Part model, mm, in its own coordinate system. Face numbers are marked on the shaded views. A direction names the side the tool comes from. Round coordinates to 2 decimals unless told otherwise and drop trailing zeros. Write each loop counter-clockwise with the first axis right and the second up, starting at its lowest first coordinate (ties: lowest second). Pieces come first, ordered by that corner, then holes. Notation, with made-up numbers: M 23.5,-11 L 52.5,-11 A27 ccw 52.5,16 Z; hole C 59,80.5 d2. An arc over 180 degrees is marked long. One line per question, with ' | ' between items. Start each with the question number.
1) Drop flat-ended pins along their axis: pin 1 Ø1.5 at (y, z) = (4.5, 2.5) entering from +X; pin 2 Ø0.7 at (y, z) = (-5, 1.5) entering from +X; pin 3 Ø1 at (x, y) = (2.5, -0.5) entering from -Z. Give the stop position or say it passes through.
2) Mould opens along Y. For the marked faces 1, 2, 3 and 4 say: pulls with the +Y half, pulls with the -Y half, needs draft (parallel to the pull), parting line crosses it, or undercut.
3) Saw through at A-A (z = 1.3). List the corners of the cut face in (x, y) (3 decimals), plus the area to 3 significant figures.
4) Saw through at B-B (z = 2.4). List the corners of the cut face in (x, y) (3 decimals), plus the area to 3 significant figures.
5) Wall check: probe 1 along Y at (x, z) = (4.5, 2.75); probe 2 along X at (y, z) = (-0.5, 3.05); probe 3 along Y at (x, z) = (-0.75, 3.2). Give the ranges that are in metal, low to high. Write a range as [from, to].
6) Saw through at D-D (z = 0.25). List the corners of the cut face in (x, y) (3 decimals), plus the area to 3 significant figures.
7) Tool access for the marked faces 5, 6, 7 and 8: list every direction of +Z, -Z, +X, -X, +Y, -Y with a clear straight run to the whole face (end or side of a thin tool).
8) Saw through at C-C (x = 5). List the corners of the cut face in (y, z), plus the area to 3 significant figures.
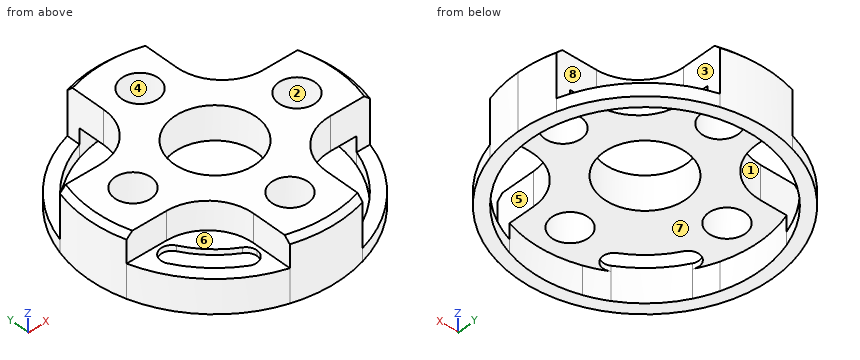
```python
from build123d import *
from build123d import SkipClean  # not in build123d's __all__

# Parameters (mm, degrees)
F0_R     = 1
F0_R_2   = 2.25
F1_DEPTH = 3.4
F2_DEPTH = 0.7
F3_DEPTH = 1.85
F4_DEPTH = 1.55
F5_R     = 2.5
F6_SIZE  = 0.3
F8_DEPTH = 1.851


# Not quite as in the source:
# - after a boolean that leaves OpenCascade's solid faulty, fix() repairs it


with BuildPart() as f1:
    # F0 (on Top) → F1 (new body)
    with BuildSketch(Plane.XY):
        with BuildLine():
            Line((2, 5.9477411679), (2, 6.6821123157))
            ThreePointArc((2, 6.6821123157), (0, 6.975), (-2, 6.6821123157))
            Line((-2, 6.6821123157), (-2, 5.9477411679))
            ThreePointArc((-2, 5.9477411679), (0, 6.275), (2, 5.9477411679))
        make_face()
        with BuildLine():
            ThreePointArc((6.275, 0), (6.1926448642, 1.013298863), (5.9477411679, 2))
            Line((5.9477411679, 2), (2, 2))
            Line((2, 2), (2, 5.9477411679))
            ThreePointArc((2, 5.9477411679), (0, 6.275), (-2, 5.9477411679))
            Line((-2, 5.9477411679), (-2, 2))
            Line((-2, 2), (-5.9477411679, 2))
            ThreePointArc((-5.9477411679, 2), (-6.275, 0), (-5.9477411679, -2))
            Line((-5.9477411679, -2), (-2, -2))
            Line((-2, -2), (-2, -5.9477411679))
            ThreePointArc((-2, -5.9477411679), (0, -6.275), (2, -5.9477411679))
            Line((2, -5.9477411679), (2, -2))
            Line((2, -2), (5.9477411679, -2))
            ThreePointArc((5.9477411679, -2), (6.1926448642, -1.013298863), (6.275, 0))
        make_face()
        with Locations((0, -4.5)):
            Circle(F0_R, mode=Mode.SUBTRACT)
        with Locations((-4.5, 0)):
            Circle(F0_R, mode=Mode.SUBTRACT)
        Circle(F0_R_2, mode=Mode.SUBTRACT)
        with Locations((4.5, 0)):
            Circle(F0_R, mode=Mode.SUBTRACT)
        with Locations((0, 4.5)):
            Circle(F0_R, mode=Mode.SUBTRACT)
        with BuildLine():
            ThreePointArc((6.6821123157, -2), (6.9013896572, -1.0106660175), (6.975, 0))
            ThreePointArc((6.975, 0), (6.9013896572, 1.0106660175), (6.6821123157, 2))
            Line((6.6821123157, 2), (5.9477411679, 2))
            ThreePointArc((5.9477411679, 2), (6.1926448642, 1.013298863), (6.275, 0))
            ThreePointArc((6.275, 0), (6.1926448642, -1.013298863), (5.9477411679, -2))
            Line((5.9477411679, -2), (6.6821123157, -2))
        make_face()
        with BuildLine():
            Line((-5.9477411679, 2), (-6.6821123157, 2))
            ThreePointArc((-6.6821123157, 2), (-6.975, 0), (-6.6821123157, -2))
            Line((-6.6821123157, -2), (-5.9477411679, -2))
            ThreePointArc((-5.9477411679, -2), (-6.275, 0), (-5.9477411679, 2))
        make_face()
        with BuildLine():
            ThreePointArc((-2, -6.6821123157), (0, -6.975), (2, -6.6821123157))
            Line((2, -6.6821123157), (2, -5.9477411679))
            ThreePointArc((2, -5.9477411679), (0, -6.275), (-2, -5.9477411679))
            Line((-2, -5.9477411679), (-2, -6.6821123157))
        make_face()
    extrude(amount=F1_DEPTH)

    # F0 (on Top) → F2 (join)
    with BuildSketch(Plane.XY):
        with BuildLine():
            Line((-2, 5.9477411679), (-2, 6.6821123157))
            ThreePointArc((-2, 6.6821123157), (-4.9320697988, 4.9320697988), (-6.6821123157, 2))
            Line((-6.6821123157, 2), (-5.9477411679, 2))
            ThreePointArc((-5.9477411679, 2), (-4.4370950519, 4.4370950519), (-2, 5.9477411679))
        make_face()
        with BuildLine():
            Line((5.9477411679, 2), (6.6821123157, 2))
            ThreePointArc((6.6821123157, 2), (4.9320697988, 4.9320697988), (2, 6.6821123157))
            Line((2, 6.6821123157), (2, 5.9477411679))
            ThreePointArc((2, 5.9477411679), (4.4370950519, 4.4370950519), (5.9477411679, 2))
        make_face()
        with BuildLine():
            ThreePointArc((2, -6.6821123157), (4.9320697988, -4.9320697988), (6.6821123157, -2))
            Line((6.6821123157, -2), (5.9477411679, -2))
            ThreePointArc((5.9477411679, -2), (4.4370950519, -4.4370950519), (2, -5.9477411679))
            Line((2, -5.9477411679), (2, -6.6821123157))
        make_face()
    extrude(amount=F2_DEPTH)

    # F0 (on Top) → F3 (join, through all)
    with BuildSketch(Plane.XY):
        with BuildLine():
            ThreePointArc((-5.9477411679, -2), (-4.4370950519, -4.4370950519), (-2, -5.9477411679))
            Line((-2, -5.9477411679), (-2, -2))
            Line((-2, -2), (-5.9477411679, -2))
        make_face()
        with BuildLine():
            ThreePointArc((-6.6821123157, -2), (-4.9320697988, -4.9320697988), (-2, -6.6821123157))
            Line((-2, -6.6821123157), (-2, -5.9477411679))
            ThreePointArc((-2, -5.9477411679), (-4.4370950519, -4.4370950519), (-5.9477411679, -2))
            Line((-5.9477411679, -2), (-6.6821123157, -2))
        make_face()
    extrude(amount=F3_DEPTH)

    # F0 (on Top) → F4 (cut, through all)
    with BuildSketch(Plane.XY):
        with BuildLine():
            ThreePointArc((6.275, 0), (6.1926448642, 1.013298863), (5.9477411679, 2))
            Line((5.9477411679, 2), (2, 2))
            Line((2, 2), (2, 5.9477411679))
            ThreePointArc((2, 5.9477411679), (0, 6.275), (-2, 5.9477411679))
            Line((-2, 5.9477411679), (-2, 2))
            Line((-2, 2), (-5.9477411679, 2))
            ThreePointArc((-5.9477411679, 2), (-6.275, 0), (-5.9477411679, -2))
            Line((-5.9477411679, -2), (-2, -2))
            Line((-2, -2), (-2, -5.9477411679))
            ThreePointArc((-2, -5.9477411679), (0, -6.275), (2, -5.9477411679))
            Line((2, -5.9477411679), (2, -2))
            Line((2, -2), (5.9477411679, -2))
            ThreePointArc((5.9477411679, -2), (6.1926448642, -1.013298863), (6.275, 0))
        make_face()
        with Locations((0, -4.5)):
            Circle(F0_R, mode=Mode.SUBTRACT)
        with Locations((-4.5, 0)):
            Circle(F0_R, mode=Mode.SUBTRACT)
        Circle(F0_R_2, mode=Mode.SUBTRACT)
        with Locations((4.5, 0)):
            Circle(F0_R, mode=Mode.SUBTRACT)
        with Locations((0, 4.5)):
            Circle(F0_R, mode=Mode.SUBTRACT)
        with BuildLine():
            ThreePointArc((-5.9477411679, -2), (-4.4370950519, -4.4370950519), (-2, -5.9477411679))
            Line((-2, -5.9477411679), (-2, -2))
            Line((-2, -2), (-5.9477411679, -2))
        make_face()
    with SkipClean():  # cleaning this boolean's faces spoils the solid; the shape is the same uncleaned
        extrude(amount=F4_DEPTH, mode=Mode.SUBTRACT)

    # F5
    f5_edges = [f1.edges().sort_by_distance(p)[0] for p in [
        (-2, 2, 2.475),
        (-2, -2, 2.625),
        (2, -2, 2.475),
        (2, 2, 2.475),
    ]]
    fillet(f5_edges, radius=F5_R)

    # F6
    f6_edges = [f1.edges().sort_by_distance(p)[0] for p in [
        (0, -6.975, 3.4),
        (6.975, 0, 3.4),
        (0, 6.975, 3.4),
        (-6.975, 0, 3.4),
    ]]
    chamfer(f6_edges, length=F6_SIZE)

    # F7 (on face) → F8 (cut, through all)
    with BuildSketch(Plane.XY.offset(1.85)):
        with BuildLine():
            ThreePointArc((-5.4520938065, -3.106492898), (-4.777137974, -3.3894531711), (-4.330778064, -2.8094577205))
            ThreePointArc((-4.330778064, -2.8094577205), (-4.3507826134, -2.6558176305), (-4.4094623216, -2.512422543))
            ThreePointArc((-4.4094623216, -2.512422543), (-5.2278132415, -2.288141978), (-5.4520938065, -3.106492898))
        make_face()
        with BuildLine():
            ThreePointArc((-4.4094623216, -2.512422543), (-4.3507826134, -2.6558176305), (-4.330778064, -2.8094577205))
            ThreePointArc((-4.330778064, -2.8094577205), (-4.777137974, -3.3894531711), (-5.4520938065, -3.106492898))
            ThreePointArc((-5.4520938065, -3.106492898), (-4.4370950519, -4.4370950519), (-3.106492898, -5.4520938065))
            ThreePointArc((-3.106492898, -5.4520938065), (-3.3307734629, -4.6337428865), (-2.512422543, -4.4094623216))
            ThreePointArc((-2.512422543, -4.4094623216), (-3.5885669145, -3.5885669145), (-4.4094623216, -2.512422543))
        make_face()
        with BuildLine():
            ThreePointArc((-2.2094577205, -4.930778064), (-2.2906990548, -4.6292992974), (-2.512422543, -4.4094623216))
            ThreePointArc((-2.512422543, -4.4094623216), (-3.3307734629, -4.6337428865), (-3.106492898, -5.4520938065))
            ThreePointArc((-3.106492898, -5.4520938065), (-2.5079789538, -5.4495367298), (-2.2094577205, -4.930778064))
        make_face()
    extrude(amount=-F8_DEPTH, mode=Mode.SUBTRACT)

    add(f1.part.fix(), mode=Mode.REPLACE)


solid = f1.part
```
Answer key:
1) pin 1: stops at x = 2.12 | pin 2: stops at x = 2 | pin 3: stops at z = 1.55
2) face 1: pulls with the +Y half | face 2: undercut | face 3: needs draft | face 4: undercut
3) outline: M -6.682,2 A6.975 ccw 2,-6.682 L 2,-5.948 A6.275 cw -5.948,2 Z; M -2,5.948 A6.275 cw 2,5.948 L 2,6.682 A6.975 ccw -2,6.682 Z; M 5.948,-2 L 6.682,-2 A6.975 ccw 6.682,2 L 5.948,2 A6.275 cw Z | area: 15.8 mm2
4) outline: M -6.682,-2 L -4.5,-2 A2.5 cw -2,-4.5 L -2,-6.682 A6.975 ccw 2,-6.682 L 2,-4.5 A2.5 cw 4.5,-2 L 6.682,-2 A6.975 ccw 6.682,2 L 4.5,2 A2.5 cw 2,4.5 L 2,6.682 A6.975 ccw -2,6.682 L -2,4.5 A2.5 cw -4.5,2 L -6.682,2 A6.975 ccw Z; hole C -4.5,0 d2; hole C 0,0 d4.5; hole C 0,-4.5 d2; hole C 0,4.5 d2; hole C 4.5,0 d2 | area: 70.9 mm2
5) probe 1: y = [-2, -1], [1, 2] | probe 2: x = [-6.96, -5.37], [-3.63, -2.19], [2.19, 3.63], [5.37, 6.96] | probe 3: y = [-6.83, -5.16], [-3.84, -2.12], [2.12, 3.84], [5.16, 6.83]
6) outline: C 0,0 d13.95; hole C 0,0 d12.55 | area: 29.1 mm2
7) face 5: +Z, +X, -Y | face 6: +Z, -X, -Y | face 7: -Z | face 8: +Z, +X, +Y
8) outline: M -4.86,0 L -3.79,0 L -3.79,0.7 L -4.86,0.7 Z; M -2,1.55 L -0.87,1.55 L -0.87,3.4 L -2,3.4 Z; M 0.87,1.55 L 2,1.55 L 2,3.4 L 0.87,3.4 Z; M 3.79,0 L 4.86,0 L 4.86,0.7 L 3.79,0.7 Z | area: 5.70 mm2
